Study the drawing (mm; zero at the part's minimum x, y, z) and answer. Coordinates: 2 decimals unless noted, no trailing zeros. Write each loop counter-clockwise with the first axis right and the second up, starting at its lowest first coordinate (ties: lowest second). Pieces come first, ordered by that corner, then holes. Notation, with made-up numbers: M 78,10 L 107,10 A8 ccw 107,25 Z; hole C 28.25,41 d5. An arc over 180 degrees is marked long. Answer as a JSON object with one key per item and string values. Group by question number.
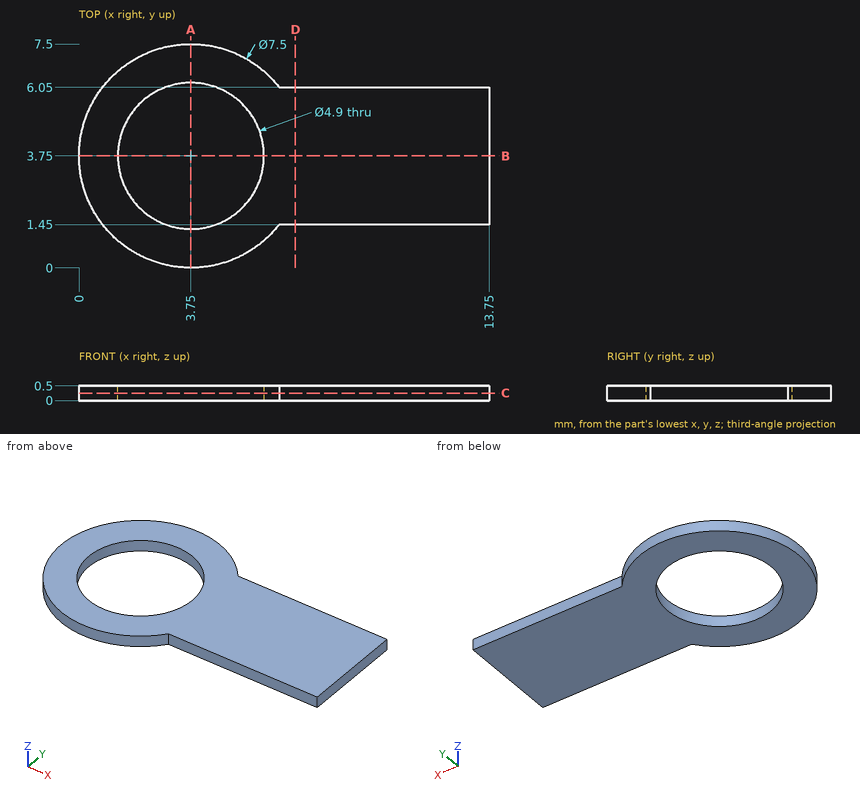
Item 1: Consider L1, parallel to Y at x = 3.75, z = 0.15; L2, parallel to Y at x = 13, z = 0.25; L3, parallel to Y at x = 4.75, z = 0.2. Determine where each line is inside the solid, lowest interval first. Write a range as from..to.
Item 2: A cutting plane is placed at D-D, the plane x = 7.25. Write down the section's boundary in (y, z), and give its area (3 significant figures).
Item 3: A cutting plane is placed at C-C, the plane z = 0.25. Write down the section's boundary in (x, y), and give its area (3 significant figures).
Item 4: A cutting plane is placed at A-A, the plane x = 3.75. Write down the section's boundary in (y, z).
Item 5: A cutting plane is placed at B-B, the plane y = 3.75. Write down the section's boundary in (x, z).
Answer:
{
 "1": {"L1": "0..1.3, 6.2..7.5", "L2": "1.45..6.05", "L3": "0.14..1.51, 5.99..7.36"},
 "2": {"outline": "M 1.45,0 L 6.05,0 L 6.05,0.5 L 1.45,0.5 Z", "area": "2.30 mm2"},
 "3": {"outline": "M 6.71,1.45 L 13.75,1.45 L 13.75,6.05 L 6.71,6.05 A3.75 ccw long Z; hole C 3.75,3.75 d4.9", "area": "55.2 mm2"},
 "4": {"outline": "M 0,0 L 1.3,0 L 1.3,0.5 L 0,0.5 Z; M 6.2,0 L 7.5,0 L 7.5,0.5 L 6.2,0.5 Z"},
 "5": {"outline": "M 0,0 L 1.3,0 L 1.3,0.5 L 0,0.5 Z; M 6.2,0 L 13.75,0 L 13.75,0.5 L 6.2,0.5 Z"}
}
